```python
from build123d import *

# Parameters (mm, degrees)
F1_DEPTH       = 207.9847365
F2_T1_DEPTH    = 312.4469684912
F3_T1_DEPTH    = 284.4287008275
F6_START       = -2
F6_DEPTH       = 4
F9_START       = 2
F9_DEPTH       = 4
F11_R          = 20
F12_DEPTH      = 90
F12_DEPTH_BACK = 5
F13_T4_DEPTH   = 46.8692709023
F13_T9_DEPTH   = 46.8692709023


# Not quite as in the source:
# - a fillet or chamfer that OpenCascade refuses, or shapes differently, is made with other operations: its cross-section is extruded or revolved along the edge and cut away or added


with BuildPart() as f1:
    # F0 (on Front) → F1 (new body)
    with BuildSketch(Plane.XZ):
        with BuildLine():
            Line((-18, 0), (0, 0))
            Line((0, 0), (18, 0))
            ThreePointArc((18, 0), (18.2679491924, 1), (18, 2))
            Line((18, 2), (16, 2))
            ThreePointArc((16, 2), (13.9795897113, 22), (16, 42))
            Line((16, 42), (19, 42))
            ThreePointArc((19, 42), (19.4019237886, 43.5), (19, 45))
            ThreePointArc((19, 45), (0, 48.7506756806), (-19, 45))
            ThreePointArc((-19, 45), (-19.4019237886, 43.5), (-19, 42))
            Line((-19, 42), (-16, 42))
            ThreePointArc((-16, 42), (-13.9795897113, 22), (-16, 2))
            Line((-16, 2), (-18, 2))
            ThreePointArc((-18, 2), (-18.2679491924, 1), (-18, 0))
        make_face()
        with BuildLine():
            Line((14, 3), (0, 3))
            Line((0, 3), (-14, 3))
            ThreePointArc((-14, 3), (-11.9795897113, 23), (-14, 43))
            ThreePointArc((-14, 43), (0, 45), (14, 43))
            ThreePointArc((14, 43), (11.9795897113, 23), (14, 3))
        make_face(mode=Mode.SUBTRACT)
    extrude(amount=F1_DEPTH)

    # F2: chamfer of 45 x 53.6289116667 on 1 edges, made by hand

    # F2_s2 → F2_t1 (cut)
    with BuildSketch(Plane.YZ.offset(-156.2234842456)):
        Polygon((-207.9847365, 53.6289116667), (-162.9847365, 0), (-207.9847365, 0), align=None)
    extrude(amount=F2_T1_DEPTH, mode=Mode.SUBTRACT)

    # F3: chamfer of 45 x 48.2565919511 on 1 edges, made by hand

    # F3_s2 → F3_t1 (cut)
    with BuildSketch(Plane.YZ.offset(-142.2143504137)):
        Polygon((0, 45), (-48.2565919511, 0), (0, 0), align=None)
    extrude(amount=F3_T1_DEPTH, mode=Mode.SUBTRACT)

    # F5 (on face) → F6 (cut)
    with BuildSketch(Plane(origin=(14, 0, 0), x_dir=(0, -1, 0), z_dir=(-1, 0, 0)).offset(F6_START)):
        Polygon((200.7156460232, 72.1911139462), (140.1401089367, 0), (198.049341578, 0), (232.2688040982, 72.1911139462), align=None)
    extrude(amount=-F6_DEPTH, mode=Mode.SUBTRACT)

    # F8 (on face) → F9 (cut)
    with BuildSketch(Plane(origin=(-14, 0, 0), x_dir=(0, -1, 0), z_dir=(-1, 0, 0)).offset(F9_START)):
        Polygon((185.9322765967, 54.5729803215), (140.1401089367, 0), (168.9397689519, 0), (210.618345394, 54.5729803215), align=None)
    extrude(amount=F9_DEPTH, mode=Mode.SUBTRACT)

    # F11 (on face) → F12 (cut, two sides)
    with BuildSketch(Plane(origin=(0, 22.4451911308, 20.9304793408), x_dir=(-1, 0, 0), z_dir=(0, 0.7313537016, 0.6819983601))) as f12_sk:
        with Locations((0, 26.6659185749)):
            Circle(F11_R)
    extrude(amount=-F12_DEPTH, mode=Mode.SUBTRACT)
    extrude(f12_sk.sketch, amount=F12_DEPTH_BACK, mode=Mode.SUBTRACT)

    # F13: fillet of radius 6 on 2 edges, made by hand


with BuildPart() as f13_tool2:
    # F13_s3 → F13_t4 (new body)
    with BuildSketch(Plane.XZ.offset(213.6976361216)):
        with BuildLine():
            ThreePointArc((11.3791048339, 47.4386205251), (14.5860497205, 45.4810144553), (16, 42))
            Line((16, 42), (16, 46.1215528099))
            ThreePointArc((16, 46.1215528099), (13.7053826002, 46.8356264218), (11.3791048339, 47.4386205251))
        make_face()
    extrude(amount=-F13_T4_DEPTH)

    split(bisect_by=Plane(origin=(0, -82.2375917358, -69.0055328944), x_dir=(1, 0, 0), z_dir=(0, -0.7660444431, -0.6427876097)), keep=Keep.TOP)


with BuildPart() as f1_1:
    add(f1.part)

    # F13_t1: cut F13_tool2
    add(f13_tool2.part, mode=Mode.SUBTRACT)


with BuildPart() as f13_tool7:
    # F13_s8 → F13_t9 (new body)
    with BuildSketch(Plane.XZ.offset(213.6976361216)):
        with BuildLine():
            ThreePointArc((-16, 42), (-14.5860497205, 45.4810144553), (-11.3791048339, 47.4386205251))
            ThreePointArc((-11.3791048339, 47.4386205251), (-13.7053826002, 46.8356264218), (-16, 46.1215528099))
            Line((-16, 46.1215528099), (-16, 42))
        make_face()
    extrude(amount=-F13_T9_DEPTH)

    split(bisect_by=Plane(origin=(0, -82.2375917358, -69.0055328944), x_dir=(1, 0, 0), z_dir=(0, -0.7660444431, -0.6427876097)), keep=Keep.TOP)


with BuildPart() as f1_2:
    add(f1_1.part)

    # F13_t6: cut F13_tool7
    add(f13_tool7.part, mode=Mode.SUBTRACT)


solid = f1_2.part
```
The listing builds one solid part. Answer for the finished solid, in the listing's coordinates (mm). A direction names the side the tool comes from. Coordinates: 2 decimals unless noted, no trailing zeros. Loops run counter-clockwise (first coordinate to the right, second up) from the corner with the lowest first, then second, coordinate; pieces in that order, holes last. Notation, with made-up numbers: M -11,15.5 L 45,15.5 A27 ccw 45,51.5 Z; hole C -6.5,-8.5 d9. An arc over 180 degrees is marked long. Answer as a JSON object with one key per item and string values. Group by question number.
Item 1: Section A-A (y = -104) is taken. Write down the section's boundary in (x, z), and give its area (3 significant figures).
Item 2: Section C-C (y = -169.5) is taken. Write down the section's boundary in (x, z), and give its area (3 significant figures).
Item 3: Determine the mould class of faces 3 (the face through (0, -107, 0)), 4 (the face through (-13.98, -103.64, 22.28)), 5 (the face through (-12.19, -35.98, 24.59)) for opening direction X: +X half, -X half, draft (parallel to the pull), parting line (faces both ways), or undercut.
Item 4: Which of the six approach directions +Z, -Z, +X, -X, +Y, -Y give full straight-line access (tool end or side, diameter ignored) to faces 1 (the face through (0, -106, 45)), 2 (the face through (0.27, -100.63, 48.75))?
Item 5: Each of these flat-tipped pins is pushed along its axis until it touches: P1, Ø8, axis at y = -98, z = 27, coming from the +X side; P2, Ø12, axis at x = 14, z = 35.5, coming from the -Y side; P3, Ø6, axis at x = 8.5, z = 32, coming from the +Y side; P4, Ø6, axis at x = -14, z = 10.5, coming from the -Y side. Where does it stop, or does it pass through?
Item 6: Section D-D (x = 6.5) is taken. Write down the section's boundary in (y, z), and give its area (3 significant figures).
Item 7: Section B-B (x = -2) is taken. Write down the section's boundary in (y, z), and give its area (3 significant figures).
Item 8: Consider L1, parallel to X at y = -76.5, z = 20.5; L2, parallel to Z at x = 4, y = -148; L3, parallel to Z at x = 9.5, y = -112. Determine where each line is inside the solid, lowest interval first.
Solved:
{
 "1": {"outline": "M -19,42 L -16,42 A100 cw -16,2 L -18,2 A2 ccw -18,0 L 18,0 A2 ccw 18,2 L 16,2 A100 cw 16,42 L 19,42 A3 ccw 19,45 A50 ccw -19,45 A3 ccw Z; hole M -14,3 L 14,3 A100 cw 14,43 A50 ccw -14,43 A100 cw Z", "area": "407 mm2"},
 "2": {"outline": "M -19,42 L -16,42 A100 cw -15,7.76 L -13.15,7.76 A100 ccw -14,43 A50 cw 14,43 A100 ccw 13.15,7.76 L 15,7.76 A100 cw 16,42 L 19,42 A3 ccw 19,45 A50 ccw -19,45 A3 ccw Z", "area": "285 mm2"},
 "3": {"face 3": "draft", "face 4": "-X half", "face 5": "undercut"},
 "4": {"face 1": "+Y, -Y", "face 2": "+Z, +Y, -Y"},
 "5": {"P1": "stops at x = 14.39", "P2": "stops at y = -197.81", "P3": "passes through", "P4": "stops at y = -174.31"},
 "6": {"outline": "M -203.54,48.33 L -200.39,44.58 L -19.03,44.58 L -15.01,48.33 Z; M -165.5,3 L -162.98,0 L -66.83,0 L -63.62,3 Z", "area": "991 mm2"},
 "7": {"outline": "M -203.86,48.71 L -200.71,44.96 L -20.06,44.96 L -16.04,48.71 Z; M -165.5,3 L -162.98,0 L -68.28,0 L -65.06,3 Z", "area": "984 mm2"},
 "8": {"L1": "x = -13.99 to -12.01, 12.01 to 13.99", "L2": "z = 0 to 3, 44.84 to 48.59", "L3": "z = 0 to 3, 44.09 to 47.84"}
}
